The model under review builds one solid part; all positions refer to its coordinate system, in mm. Round coordinates to 2 decimals unless told otherwise and drop trailing zeros. Order: outer loops, then holes, each group sorted by start corner. A loop starts at its lowest first (then second) coordinate and runs counter-clockwise, first axis right, second up. Notation, with made-up numbers: (77.25, 45) -> (123.25, 45) arc R18 cw to (123.25, 60) -> close; hole circle Ø6 at (10.5, 7). An arc over 180 degrees is marked (long way). Use a Markdown table: item, result. Add a question column.
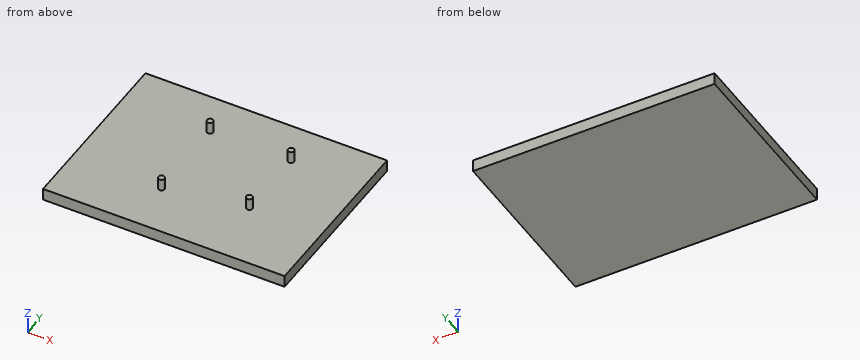
```python
from build123d import *

# Parameters (mm, degrees)
F0_W       = 508
F0_H       = 381
F1_DEPTH   = 25.4
F2_R       = 6.35
F3_DEPTH   = 25.4
F1_FACE1_W = 508
F1_FACE1_H = 381
F4_DEPTH   = 25.4
F5_DEPTH   = 25.4


# Not quite as in the source:
# - a feature names something its author has since deleted; it is built from what else it names


with BuildPart() as f1:
    # F0 (on Top) → F1 (new body)
    with BuildSketch(Plane.XY):
        with Locations((15.942402184, 51.6951617887)):
            Rectangle(F0_W, F0_H)
    extrude(amount=F1_DEPTH)

    # F2 (on face) → F3 (join)
    with BuildSketch(Plane.XY.offset(25.4)):
        with Locations((-52.637597816, 154.94)):
            Circle(F2_R)
        with Locations((117.542402184, 154.94)):
            Circle(F2_R)
        with Locations((117.542402184, 0)):
            Circle(F2_R)
    extrude(amount=F3_DEPTH)

    # F2 (on face) + F1_face1 (on face) → F4 (join)
    with BuildSketch(Plane.XY.offset(25.4)):
        with Locations((-52.637597816, 154.94)):
            Circle(F2_R)
        with Locations((117.542402184, 154.94)):
            Circle(F2_R)
        with Locations((117.542402184, 0)):
            Circle(F2_R)
        with Locations((-50.097597816, -30.48)):
            Circle(F2_R)
    with BuildSketch(Plane(origin=(15.942402184, 51.6951617887, 0), x_dir=(1, 0, 0), z_dir=(0, 0, -1))):
        Rectangle(F1_FACE1_W, F1_FACE1_H)
    extrude(amount=F4_DEPTH, dir=(0, 0, 1))

    # F2 (on face) + F1_face1 (on face) → F5 (join)
    with BuildSketch(Plane.XY.offset(25.4)):
        with Locations((-52.637597816, 154.94)):
            Circle(F2_R)
        with Locations((117.542402184, 154.94)):
            Circle(F2_R)
        with Locations((117.542402184, 0)):
            Circle(F2_R)
        with Locations((-50.097597816, -30.48)):
            Circle(F2_R)
    with BuildSketch(Plane(origin=(15.942402184, 51.6951617887, 0), x_dir=(1, 0, 0), z_dir=(0, 0, -1))):
        Rectangle(F1_FACE1_W, F1_FACE1_H)
    extrude(amount=F5_DEPTH, dir=(0, 0, 1))


solid = f1.part
```
Q1. Wall thickness on line 1 (Z direction, x = 16.5, y = -0.5); line 2 (X direction, y = 3, z = 33): over which ranges is each line inside the solid? List them lowest first. Write a range as [from, to].
Q2. Add section B-B (x = 193). Write out the cut boundary in (y, z), then the cut area to 3 significant figures.
Q3. Add section D-D (y = 93.5). Write out the cut boundary in (x, z), then the cut area to 3 significant figures.
Q4. Insertion check: pin 1 (1 mm diameter, centred on x = 120, z = 28.5, fed in from -Y); pin 2 (1 mm diameter, centred on y = -8.5, z = 26, fed in from -X); pin 3 (1 mm diameter, centred on y = 4.5, z = 32, fed in from +X). Each pin has a flat end and moves straight along its axis. Give the tip position at first contact, or say it passes through.
Q5. Add section C-C (y = -30.48). Write out the cut boundary in (x, z).
Q6. Add section A-A (y = 154.94). Write out the cut boundary in (x, z).
Report:
| question | item | result |
|---|---|---|
| 1 | line 1 | z = [0, 25.4] |
| 1 | line 2 | x = [111.95, 123.14] |
| 2 | outline | (-138.8, 0) -> (242.2, 0) -> (242.2, 25.4) -> (-138.8, 25.4) -> close |
| 2 | area | 9,680 mm² |
| 3 | outline | (-238.06, 0) -> (269.94, 0) -> (269.94, 25.4) -> (-238.06, 25.4) -> close |
| 3 | area | 12,900 mm² |
| 4 | pin 1 | stops at y = -6.04 |
| 4 | pin 2 | passes through |
| 4 | pin 3 | stops at x = 122.47 |
| 5 | outline | (-238.06, 0) -> (269.94, 0) -> (269.94, 25.4) -> (-43.75, 25.4) -> (-43.75, 50.8) -> (-56.45, 50.8) -> (-56.45, 25.4) -> (-238.06, 25.4) -> close |
| 6 | outline | (-238.06, 0) -> (269.94, 0) -> (269.94, 25.4) -> (123.89, 25.4) -> (123.89, 50.8) -> (111.19, 50.8) -> (111.19, 25.4) -> (-46.29, 25.4) -> (-46.29, 50.8) -> (-58.99, 50.8) -> (-58.99, 25.4) -> (-238.06, 25.4) -> close |
